Verification items for this drawing (mm, ordinates from the low corner). A direction names the side the tool comes from. Give positions to 0.01 mm unless a question says otherwise; leave off trailing zeros. Loops run counter-clockwise (first coordinate to the right, second up) from the corner with the lowest first, then second, coordinate; pieces in that order, holes last. Notation, with made-up numbers: (76.5, 39.25) - (111.5, 39.25) arc R32 ccw to (111.5, 71.25) - close; hole circle Ø3 at (9, 6). An arc over 180 degrees is marked (long way). One line per question, with ' | ' between items. Start each with the question number.
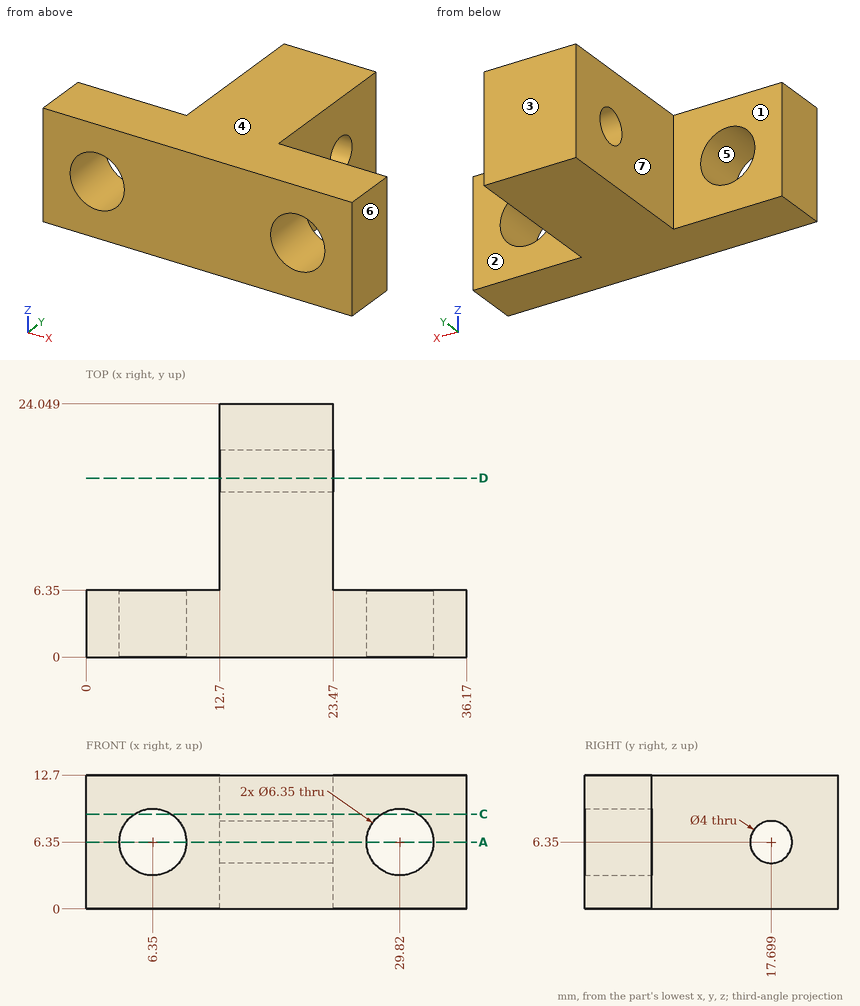
(1) Mould release check, pull along X, two halves, no side actions. Record for the marked faces 4, 5, 6 and 7: pulls with the +X half, pulls with the -X half, needs draft (parallel to the pull), parting line crosses it, or undercut.
(2) Section check A-A, the plane z = 6.35. Count the separate pieces of the cut face and the enclosed holes in it.
(3) Section check C-C, the plane z = 9. Record the boundary of the cut face in (x, y), and give its area (3 significant figures).
(4) Material ranges on line 1 (X direction, y = 1.75, z = 6.35) (1 decimal); line 2 (Z direction, x = 6.35, y = 4.75) (1 decimal); line 3 (X direction, y = 3.75, z = 4.25), recorded low to high.
(5) Section check D-D, the plane y = 17. Record the boundary of the cut face in (x, z).
(6) Depth check by flat-ended pin: pin 1 Ø4.5 at (y, z) = (17.699, 6.35) entering from -X; pin 2 Ø4 at (x, z) = (28, 4.5) entering from +Y. Enter the tip coordinate at first touch or a pass-through.
(7) Tool access check on the marked faces 1, 2 and 3. Record the directions out of +Z, -Z, +X, -X, +Y, -Y that give a thin tool (end or side, any length) a straight path to the whole face; none if there is none.
Numbers:
1) face 4: needs draft | face 5: undercut | face 6: pulls with the +X half | face 7: pulls with the -X half
2) separate pieces: 4 | enclosed holes: 0
3) outline: (0, 0) - (4.6, 0) - (4.6, 6.35) - (0, 6.35) - close; (8.1, 0) - (28.07, 0) - (28.07, 6.35) - (23.47, 6.35) - (23.47, 24.05) - (12.7, 24.05) - (12.7, 6.35) - (8.1, 6.35) - close; (31.57, 0) - (36.17, 0) - (36.17, 6.35) - (31.57, 6.35) - close | area: 376 mm^2
4) line 1: 0 to 3.2, 9.5 to 26.6, 33 to 36.2 | line 2: 0 to 3.2, 9.5 to 12.7 | line 3: 0 to 3.97, 8.73 to 27.44, 32.2 to 36.17
5) outline: (12.7, 0) - (23.47, 0) - (23.47, 4.48) - (12.7, 4.48) - close; (12.7, 8.22) - (23.47, 8.22) - (23.47, 12.7) - (12.7, 12.7) - close
6) pin 1: x = 12.7 | pin 2: y = 6.35
7) face 1: +Z, -Z, -X, +Y | face 2: +Z, -Z, +X, +Y | face 3: +Z, -Z, +X, -X, +Y
